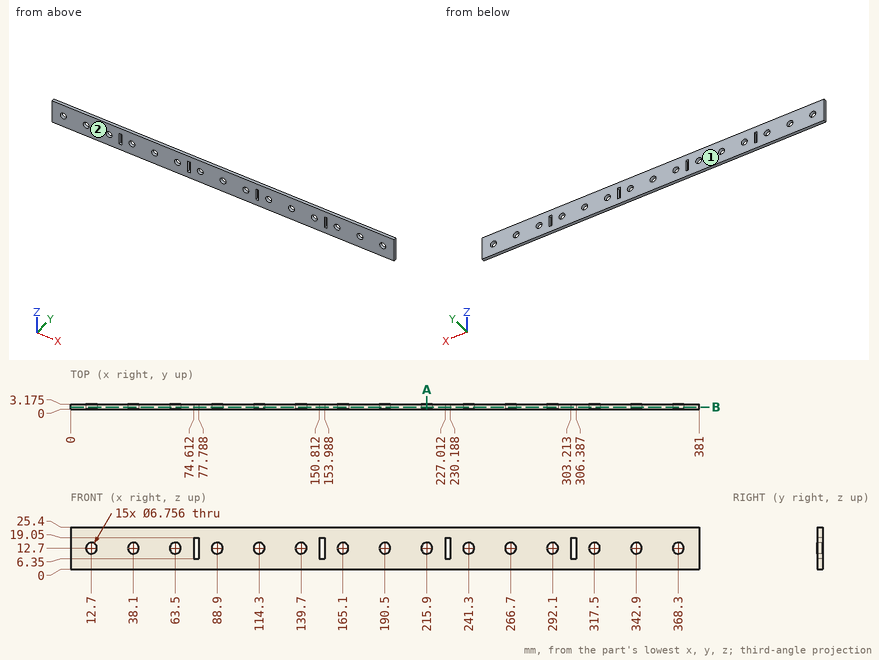
Here's the drawing with two shaded views (mm, measured from the low corner). I have some questions. Give positions to 0.01 mm unless a question says otherwise; leave off trailing zeros. Loops run counter-clockwise (first coordinate to the right, second up) from the corner with the lowest first, then second, coordinate; pieces in that order, holes last. Notation, with made-up numbers: M 2,52.5 L 23,52.5 A30 ccw 23,84.5 Z; hole C 64,-3 d6. An arc over 180 degrees is marked long. Use one line per item in the form item = value. Start each with the question number.
Q1. I need wall thicknesses on line 1 along Z through (x, y) = (88.9, 1.7); line 2 along Z through (x, y) = (91, 2.5) (1 decimal). Which ranges of each line are inside material? Lowest first, please.
Q2. If we section it at A-A (x = 215.9): Write out the boundary of the cut face in (y, z) (1 decimal).
Q3. Will this pin go through, and if not, where does the flat tip stop? pin 1 Ø5.5 at (x, z) = (88.9, 12.7) entering from -Y.
Q4. If we section it at B-B (y = 1.3): State how many separate pieces and enclosed holes the cut face has, then the cut area to 3 significant figures.
Q5. Thinking about a two-plate mould opening in Y: for the marked faces 1 and 2, which applies, +Y half, -Y half, draft (parallel to the pull), parting line (faces both ways), or undercut?
Taken from the geometry:
q1.line_1 = 0 to 9.32, 16.08 to 25.4
q1.line_2 = 0 to 10.1, 15.3 to 25.4
q2.outline = M 0,0 L 3.2,0 L 3.2,9.3 L 0,9.3 Z; M 0,16.1 L 3.2,16.1 L 3.2,25.4 L 0,25.4 Z
q3.pin_1 = through
q4.separate_pieces = 1
q4.enclosed_holes = 19
q4.area = 8,980 mm^2
q5.face_1 = +Y half
q5.face_2 = -Y half
